from build123d import *

# Parameters (mm, degrees)
F0_R     = 1
F1_DEPTH = 19.5
F2_W     = 7.5
F2_H     = 18.5
F3_DEPTH = 12.5


with BuildPart() as f1:
    # F0 (on Top) → F1 (new body)
    with BuildSketch(Plane.XY):
        with BuildLine():
            Line((30.25, 18.55), (-30.25, 18.55))
            ThreePointArc((-30.25, 18.55), (-33.078427, 17.378427), (-34.25, 14.55))
            Line((-34.25, 14.55), (-34.25, 6.5))
            Line((-34.25, 6.5), (-34.25, -6.5))
            Line((-34.25, -6.5), (-34.25, -14.55))
            ThreePointArc((-34.25, -14.55), (-33.078427, -17.378427), (-30.25, -18.55))
            Line((-30.25, -18.55), (30.25, -18.55))
            ThreePointArc((30.25, -18.55), (33.078427, -17.378427), (34.25, -14.55))
            Line((34.25, -14.55), (34.25, -6.5))
            Line((34.25, -6.5), (34.25, 6.5))
            Line((34.25, 6.5), (34.25, 14.55))
            ThreePointArc((34.25, 14.55), (33.078427, 17.378427), (30.25, 18.55))
        make_face()
        with BuildLine():
            Line((-34.25, -6.5), (-34.25, 6.5))
            Line((-34.25, 6.5), (-40.75, 6.5))
            ThreePointArc((-40.75, 6.5), (-41.457107, 6.207107), (-41.75, 5.5))
            Line((-41.75, 5.5), (-41.75, -5.5))
            ThreePointArc((-41.75, -5.5), (-41.457107, -6.207107), (-40.75, -6.5))
            Line((-40.75, -6.5), (-34.25, -6.5))
        make_face()
        with Locations((-39.75, -4)):
            Circle(F0_R, mode=Mode.SUBTRACT)
        with Locations((-39.75, 0)):
            Circle(F0_R, mode=Mode.SUBTRACT)
        with Locations((-39.75, 4)):
            Circle(F0_R, mode=Mode.SUBTRACT)
        with BuildLine():
            Line((40.75, 6.5), (34.25, 6.5))
            Line((34.25, 6.5), (34.25, -6.5))
            Line((34.25, -6.5), (40.75, -6.5))
            ThreePointArc((40.75, -6.5), (41.457107, -6.207107), (41.75, -5.5))
            Line((41.75, -5.5), (41.75, 5.5))
            ThreePointArc((41.75, 5.5), (41.457107, 6.207107), (40.75, 6.5))
        make_face()
        with Locations((39.75, -4)):
            Circle(F0_R, mode=Mode.SUBTRACT)
        with Locations((39.75, 0)):
            Circle(F0_R, mode=Mode.SUBTRACT)
        with Locations((39.75, 4)):
            Circle(F0_R, mode=Mode.SUBTRACT)
    extrude(amount=F1_DEPTH)

    # F2 (on Front) → F3 (cut, symmetric)
    with BuildSketch(Plane.XZ):
        with Locations((-38, 10.25)):
            Rectangle(F2_W, F2_H)
        with Locations((38, 10.25)):
            Rectangle(F2_W, F2_H)
    extrude(amount=F3_DEPTH, both=True, mode=Mode.SUBTRACT)


solid = f1.part
The listing builds one solid part. Answer for the finished solid, in the listing's coordinates (mm). A direction names the side the tool comes from. Coordinates: 2 decimals unless noted, no trailing zeros. Loops run counter-clockwise (first coordinate to the right, second up) from the corner with the lowest first, then second, coordinate; pieces in that order, holes last. Notation, with made-up numbers: M -14.5,-36.75 L 1.5,-36.75 A13 ccw 1.5,-13.75 Z; hole C 28.5,55.5 d2. An arc over 180 degrees is marked long. Answer in a Markdown table with one row per item.
1) Which of the six approach directions +Z, -Z, +X, -X, +Y, -Y give full straight-line access (tool end or side, diameter ignored) to faces 1 (the flat face through (-38, 0, 1)), 2 (the flat face through (38, 0, 1)), 3 (the cylindrical face through (40.704, 4.3, 0.493))?
Answers below:
| item | result |
|---|---|
| face 1 | +Z, -X, +Y, -Y |
| face 2 | +Z, +X, +Y, -Y |
| face 3 | +Z, -Z |
2) Find section B-B (x = 39.75). Determine the outline of the cut face in (y, z), then the cut area to 3 significant figures.
Answers below:
| item | result |
|---|---|
| outline | M -6.5,0 L -5,0 L -5,1 L -6.5,1 Z; M -3,0 L -1,0 L -1,1 L -3,1 Z; M 1,0 L 3,0 L 3,1 L 1,1 Z; M 5,0 L 6.5,0 L 6.5,1 L 5,1 Z |
| area | 7.00 mm^2 |
3) Find section C-C (z = 9.5). Determine the outline of the cut face in (x, y).
Answers below:
| item | result |
|---|---|
| outline | M -34.25,-14.55 A4 ccw -30.25,-18.55 L 30.25,-18.55 A4 ccw 34.25,-14.55 L 34.25,14.55 A4 ccw 30.25,18.55 L -30.25,18.55 A4 ccw -34.25,14.55 Z |
4) Find the intervals of material crossed by probe 1 along Y at (x, z) = (39.75, 0.35); probe 2 along X at (y, z) = (-4, 0.4); probe 3 along X at (y, z) = (-6, 14.75), in increasing order.
Answers below:
| item | result |
|---|---|
| probe 1 | -6.5 to -5, -3 to -1, 1 to 3, 5 to 6.5 |
| probe 2 | -41.75 to -40.75, -38.75 to 38.75, 40.75 to 41.75 |
| probe 3 | -34.25 to 34.25 |
5) Determine the mould class of faces 4 (the cylindrical face through (40.704, 0.3, 0.493)), 5 (the flat face through (0, 18.55, 10)), 6 (the cylindrical face through (40.704, -3.7, 0.493)), 7 (the cylindrical face through (-33.047, 17.409, 9.614)) for opening direction X: released by +X, released by -X, zero draft, split by the parting line, or undercut.
Answers below:
| item | result |
|---|---|
| face 4 | undercut |
| face 5 | zero draft |
| face 6 | undercut |
| face 7 | released by -X |
6) Find section A-A (y = 4). Determine the outline of the cut face in (x, z), then the cut area to 3 significant figures.
Answers below:
| item | result |
|---|---|
| outline | M -41.75,0 L -40.75,0 L -40.75,1 L -41.75,1 Z; M -38.75,0 L 38.75,0 L 38.75,1 L 34.25,1 L 34.25,19.5 L -34.25,19.5 L -34.25,1 L -38.75,1 Z; M 40.75,0 L 41.75,0 L 41.75,1 L 40.75,1 Z |
| area | 1,350 mm^2 |
7) Given pin 1 (3 mm diameter, centred on y = 4, z = 14, fed in from +X); pin 2 (1 mm diameter, centred on y = -11.5, z = 10.5, fed in from -X); pin 3 (0.5 mm diameter, centred on x = 36, z = 0.5, fed in from -Y); pin 4 (8 mm diameter, centred on x = -6.5, y = 9.5, fed in from -Z), each flat-ended and moving along its own axis, determine where each tip first touches the part or whether it passes through.
Answers below:
| item | result |
|---|---|
| pin 1 | x = 34.25 |
| pin 2 | x = -34.25 |
| pin 3 | y = -6.5 |
| pin 4 | z = 0 |
